from build123d import *

# Parameters (mm, degrees)
SKETCH1_W                                      = 58
SKETCH1_H                                      = 48.3
BOSS_EXTRUDE1_DEPTH                            = 3
CSK_FOR_M3_FLAT_HEAD_MACHINE_SCREW1_AT_2_COUNT = 2
CSK_FOR_M3_FLAT_HEAD_MACHINE_SCREW1_AT_2_PITCH = 40
CSK_FOR_M3_FLAT_HEAD_MACHINE_SCREW1_AT_3_COUNT = 2
CSK_FOR_M3_FLAT_HEAD_MACHINE_SCREW1_AT_3_PITCH = 50
CSK_FOR_M3_FLAT_HEAD_MACHINE_SCREW1_AT_4_COUNT = 2
CSK_FOR_M3_FLAT_HEAD_MACHINE_SCREW1_AT_4_PITCH = 64.031242374
SKETCH6_R                                      = 1.15
CUT_EXTRUDE1_DEPTH                             = 10


with BuildPart() as part:
    # Sketch1 → Boss-Extrude1 (new body)
    with BuildSketch(Plane(origin=(0, 0, 0), x_dir=(1, 0, 0), z_dir=(0, 1, 0))):
        Rectangle(SKETCH1_W, SKETCH1_H)
    extrude(amount=BOSS_EXTRUDE1_DEPTH)

    # Sketch3 → CSK for M3 Flat Head Machine Screw1 (revolve, cut)
    with BuildSketch(Plane(origin=(25, 3, 20), x_dir=(0, 0, 1), z_dir=(1, 0, 0))):
        Polygon((0, 0), (0, 3), (1.7, 3), (1.7, 1.65), (3.35, 0), align=None)
    csk_for_m3_flat_head_machine_screw1 = revolve(axis=Axis((25, 9.35, 20), (0, -1, 0)), mode=Mode.SUBTRACT)

    # CSK for M3 Flat Head Machine Screw1 at 2: CSK for M3 Flat Head Machine Screw1 ×2
    with Locations(*[(0, 0, -i * CSK_FOR_M3_FLAT_HEAD_MACHINE_SCREW1_AT_2_PITCH) for i in range(1, CSK_FOR_M3_FLAT_HEAD_MACHINE_SCREW1_AT_2_COUNT)]):
        add(csk_for_m3_flat_head_machine_screw1, mode=Mode.SUBTRACT)

    # CSK for M3 Flat Head Machine Screw1 at 3: CSK for M3 Flat Head Machine Screw1 ×2
    with Locations(*[(-i * CSK_FOR_M3_FLAT_HEAD_MACHINE_SCREW1_AT_3_PITCH, 0, 0) for i in range(1, CSK_FOR_M3_FLAT_HEAD_MACHINE_SCREW1_AT_3_COUNT)]):
        add(csk_for_m3_flat_head_machine_screw1, mode=Mode.SUBTRACT)

    # CSK for M3 Flat Head Machine Screw1 at 4: CSK for M3 Flat Head Machine Screw1 ×2
    with Locations(*[Vector(-0.7808688094430304, 0, -0.6246950475544243) * (i * CSK_FOR_M3_FLAT_HEAD_MACHINE_SCREW1_AT_4_PITCH) for i in range(1, CSK_FOR_M3_FLAT_HEAD_MACHINE_SCREW1_AT_4_COUNT)]):
        add(csk_for_m3_flat_head_machine_screw1, mode=Mode.SUBTRACT)

    # Sketch6 → Cut-Extrude1 (cut)
    with BuildSketch(Plane(origin=(0, 3, 0), x_dir=(1, 0, 0), z_dir=(0, 1, 0))):
        with Locations(Location((-26, 10.16, 0), (0, 0, 270))):
            Circle(SKETCH6_R)
        with Locations(Location((-13.3, 10.16, 0), (0, 0, 270))):
            Circle(SKETCH6_R)
        with Locations(Location((-13.3, -10.16, 0), (0, 0, 270))):
            Circle(SKETCH6_R)
        with Locations(Location((-26, -10.16, 0), (0, 0, 270))):
            Circle(SKETCH6_R)
    extrude(amount=-CUT_EXTRUDE1_DEPTH, mode=Mode.SUBTRACT)


solid = part.part
Part model, mm, in its own coordinate system. Round coordinates to 2 decimals unless told otherwise and drop trailing zeros. Loops run counter-clockwise (first coordinate to the right, second up) from the corner with the lowest first, then second, coordinate; pieces in that order, holes last. Notation, with made-up numbers: (73, 46.5) - (126, 46.5) arc R27 cw to (126, 72.5) - close; hole circle Ø10 at (42.25, 50.5). An arc over 180 degrees is marked (long way). Answer as a JSON object with one key per item and string values.
Item 1: Band-saw the part on B-B on z = 20. List the corners of the cut face in (x, y), plus the area to 3 significant figures.
Output:
{"outline": "(-29, 0) - (-26.7, 0) - (-26.7, 1.35) - (-28.35, 3) - (-29, 3) - close; (-23.3, 0) - (23.3, 0) - (23.3, 1.35) - (21.65, 3) - (-21.65, 3) - (-23.3, 1.35) - close; (26.7, 0) - (29, 0) - (29, 3) - (28.35, 3) - (26.7, 1.35) - close", "area": "148 mm2"}
Item 2: Pull direction X, two halves, no side cores. Call faces 1 (the face through (0, 1, 24.15)), 2 (the face through (29, 1, 0)), 3 (the face through (-27.123, 1.521, -10.409)): pulls with the +X half, pulls with the -X half, needs draft (parallel to the pull), parting line crosses it, or undercut.
Output:
{"face 1": "needs draft", "face 2": "pulls with the +X half", "face 3": "undercut"}
Item 3: Pin check, flat tips, straight feed: pin 1 (1 mm diameter, centred on x = -19.5, z = -1.5, fed in from -Y); pin 2 (3 mm diameter, centred on x = 25, z = 20, fed in from -Y); pin 3 (4 mm diameter, centred on x = 25, z = -20, fed in from +Y); pin 4 (4.5 mm diameter, centred on x = -25, z = 20, fed in from +Y). Stop position of each tip, or through.
Output:
{"pin 1": "y = 0", "pin 2": "through", "pin 3": "y = 1.65", "pin 4": "y = 1.9"}
Item 4: Band-saw the part on D-D on z = 10.16. List the corners of the cut face in (x, y), plus the area to 3 significant figures.
Output:
{"outline": "(-29, 0) - (-27.15, 0) - (-27.15, 3) - (-29, 3) - close; (-24.85, 0) - (-14.45, 0) - (-14.45, 3) - (-24.85, 3) - close; (-12.15, 0) - (29, 0) - (29, 3) - (-12.15, 3) - close", "area": "160 mm2"}
Item 5: Band-saw the part on A-A on y = 2.3. State how many separate pieces and enclosed holes the cut face has, plus the area to 3 significant figures.
Output:
{"separate pieces": "1", "enclosed holes": "8", "area": "2,700 mm2"}
Item 6: Band-saw the part on C-C on x = -13.3. List the corners of the cut face in (y, z), plus the area to 3 significant figures.
Output:
{"outline": "(0, -24.15) - (3, -24.15) - (3, -11.31) - (0, -11.31) - close; (0, -9.01) - (3, -9.01) - (3, 9.01) - (0, 9.01) - close; (0, 11.31) - (3, 11.31) - (3, 24.15) - (0, 24.15) - close", "area": "131 mm2"}
Item 7: Wall check: L1, parallel to X at y = 2.4, z = -10.16; L2, parallel to X at y = 0.8, z = -20; L3, parallel to Z at x = -14, y = 2.5. Give the ranges that are in metal, low to high.
Output:
{"L1": "-29 to -27.15, -24.85 to -14.45, -12.15 to 29", "L2": "-29 to -26.7, -23.3 to 23.3, 26.7 to 29", "L3": "-24.15 to -11.07, -9.25 to 9.25, 11.07 to 24.15"}
